Design review of the part built by this model. Coordinates are the model's own, in mm. Coordinates: 2 decimals unless noted, no trailing zeros. Write each loop counter-clockwise with the first axis right and the second up, starting at its lowest first coordinate (ties: lowest second). Pieces come first, ordered by that corner, then holes. Notation, with made-up numbers: (-0.5, -21) - (8.5, -21) arc R14 ccw to (8.5, -12) - close; hole circle Ø7 at (40, 16). An arc over 180 degrees is marked (long way). Use a Markdown table: item, result.
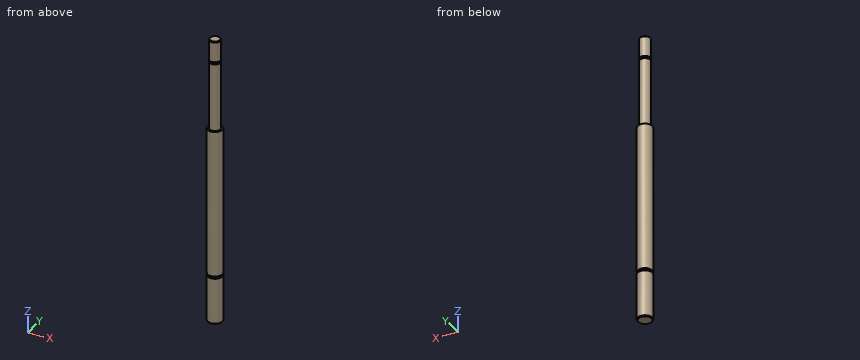
from build123d import *

# Parameters (mm, degrees)
ESQUISSE1_R          = 2
BASE_EXTRUSION_DEPTH = 54
ESQUISSE2_R          = 1.5
BOSS_EXTRU_1_DEPTH   = 25
CHANFREIN1_SIZE      = 0.2
ESQUISSE3_W          = 0.64
ESQUISSE3_H          = 2.403474903
ESQUISSE3_H_2        = 2.734022734


with BuildPart() as part:
    # Esquisse1 → Base-Extrusion (new body)
    with BuildSketch(Plane.XY):
        Circle(ESQUISSE1_R)
    extrude(amount=BASE_EXTRUSION_DEPTH)

    # Esquisse2 → Boss.-Extru.1 (add)
    with BuildSketch(Plane.XY.offset(54)):
        Circle(ESQUISSE2_R)
    extrude(amount=BOSS_EXTRU_1_DEPTH)

    # Chanfrein1
    chanfrein1_edges = [part.edges().sort_by_distance(p)[0] for p in [
        (-2, 0, 0),
        (-1.5, 0, 79),
    ]]
    chamfer(chanfrein1_edges, length=CHANFREIN1_SIZE)

    # Esquisse3 → Enlèvement de matière-Révolution1 (revolve, cut)
    with BuildSketch(Plane(origin=(0, 0, 0), x_dir=(0, 0, -1), z_dir=(1, 0, 0))):
        with Locations((-13.12, 2.801737452)):
            Rectangle(ESQUISSE3_W, ESQUISSE3_H)
        with Locations((-72.98, 2.517011367)):
            Rectangle(ESQUISSE3_W, ESQUISSE3_H_2)
    revolve(axis=Axis((0, 0, 0), (0, 0, -1)), mode=Mode.SUBTRACT)


solid = part.part
(1) Take a section at D-D on z = 72. Write out the cut boundary in (x, y), and give its area (3 significant figures).
Determined:
| item | result |
|---|---|
| outline | circle Ø3 at (0, 0) |
| area | 7.07 mm2 |
(2) Take a section at A-A on x = 0. Write out the cut boundary in (y, z), and give its area (3 significant figures).
Determined:
| item | result |
|---|---|
| outline | (-2, 0.2) - (-1.8, 0) - (1.8, 0) - (2, 0.2) - (2, 12.8) - (1.6, 12.8) - (1.6, 13.44) - (2, 13.44) - (2, 54) - (1.5, 54) - (1.5, 72.66) - (1.15, 72.66) - (1.15, 73.3) - (1.5, 73.3) - (1.5, 78.8) - (1.3, 79) - (-1.3, 79) - (-1.5, 78.8) - (-1.5, 73.3) - (-1.15, 73.3) - (-1.15, 72.66) - (-1.5, 72.66) - (-1.5, 54) - (-2, 54) - (-2, 13.44) - (-1.6, 13.44) - (-1.6, 12.8) - (-2, 12.8) - close |
| area | 290 mm2 |
(3) For L1, parallel to Z at x = -0.85, y = -0.9; L2, parallel to Z at x = 1.55, y = -0.9; L3, parallel to Y at x = -1.2, z = 40.5, list the stretches that pass through material, from the lowest coordinate up. Write a range as from..to.
Determined:
| item | result |
|---|---|
| L1 | 0..72.66, 73.3..79 |
| L2 | 0..12.8, 13.44..54 |
| L3 | -1.6..1.6 |
(4) Take a section at C-C on z = 7. Write out the cut boundary in (x, y).
Determined:
| item | result |
|---|---|
| outline | circle Ø4 at (0, 0) |
